Drawing for the job (mm, zero at the part's lowest x, y, z). A direction names the side the tool comes from. Give positions to 0.01 mm unless a question says otherwise; leave off trailing zeros. Loops run counter-clockwise (first coordinate to the right, second up) from the corner with the lowest first, then second, coordinate; pieces in that order, holes last. Notation, with made-up numbers: (38, 60.5) - (55, 60.5) arc R21 ccw to (55, 80.5) - close; hole circle Ø4 at (48, 89). An arc over 180 degrees is marked (long way). Return JSON: item names as keys, results as strings. Group by question number.
1) Drop flat-ended pins along their axis: pin 1 (5 mm diameter, centred on x = 64.5, z = 36.5, fed in from -Y); pin 2 (10.5 mm diameter, centred on y = 52.5, z = 3.5, fed in from +X); pin 3 (10.5 mm diameter, centred on y = 53, z = 46, fed in from -X); pin 4 (10.5 mm diameter, centred on x = 155, z = 13.92, fed in from +Y). Give the stop position or say it passes through.
2) Slice it at C-C (z = 13.92). List the corners of the cut face in (x, y).
3) Mould opens along Z. For the marked faces 3, 4 and 5 say: released by +Z, released by -Z, zero draft, split by the parting line, or undercut.
4) Slice it at D-D (x = 122). List the corners of the cut face in (y, z).
5) Slice it at A-A (y = 98). List the corners of the cut face in (x, z).
6) Drill centre lines: probe 1 along Z at (x, y) = (30, 6.5); probe 2 along Z at (x, y) = (98.5, 41); probe 3 along Y at (x, z) = (33.5, 41). Where is each one in solid material? Low to high. Write a range as from..to.
7) Slice it at B-B (x = 30). List the corners of the cut face in (y, z), and give its area (3 significant figures).
8) 3-axis set-ups, long thin cutter, end or side, ignore diameter. For the marked faces 1 and 2: which of +Z, -Z, +X, -X, +Y, -Y reach the whole face in a straight line?
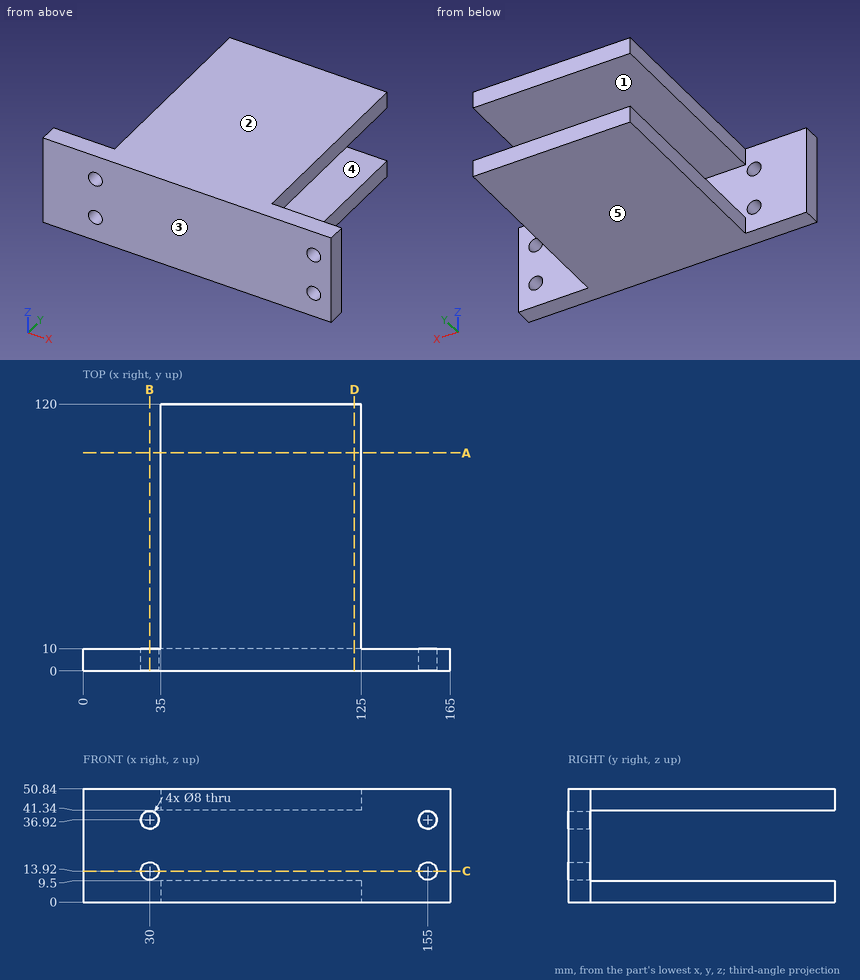
Results:
{
 "1": {"pin 1": "y = 0", "pin 2": "x = 125", "pin 3": "x = 35", "pin 4": "y = 10"},
 "2": {"outline": "(0, 0) - (26, 0) - (26, 10) - (0, 10) - close; (34, 0) - (151, 0) - (151, 10) - (34, 10) - close; (159, 0) - (165, 0) - (165, 10) - (159, 10) - close"},
 "3": {"face 3": "zero draft", "face 4": "undercut", "face 5": "released by -Z"},
 "4": {"outline": "(0, 0) - (120, 0) - (120, 9.5) - (10, 9.5) - (10, 41.34) - (120, 41.34) - (120, 50.84) - (0, 50.84) - close"},
 "5": {"outline": "(35, 0) - (125, 0) - (125, 9.5) - (35, 9.5) - close; (35, 41.34) - (125, 41.34) - (125, 50.84) - (35, 50.84) - close"},
 "6": {"probe 1": "0..9.92, 17.92..32.92, 40.92..50.84", "probe 2": "0..9.5, 41.34..50.84", "probe 3": "0..10"},
 "7": {"outline": "(0, 0) - (10, 0) - (10, 9.92) - (0, 9.92) - close; (0, 17.92) - (10, 17.92) - (10, 32.92) - (0, 32.92) - close; (0, 40.92) - (10, 40.92) - (10, 50.84) - (0, 50.84) - close", "area": "348 mm2"},
 "8": {"face 1": "+X, -X, +Y", "face 2": "+Z, +X, -X, +Y, -Y"}
}
